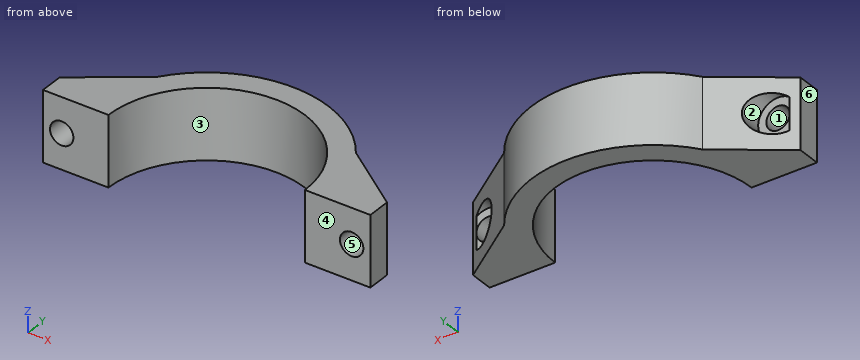
```python
from build123d import *

# Parameters (mm, degrees)
SALIENTE_EXTRUIR1_DEPTH = 7.5
SALIENTE_EXTRUIR2_DEPTH = 7.5
CROQUIS3_R              = 2.5
CORTAR_EXTRUIR1_DEPTH   = 45.240818256
CROQUIS4_R              = 4.25
CORTAR_EXTRUIR2_DEPTH   = 41.959224846


with BuildPart() as part:
    # Croquis1 → Saliente-Extruir1 (new, symmetric)
    with BuildSketch(Plane.XY):
        with BuildLine():
            Line((-26, 0), (-21, 0))
            ThreePointArc((-21, 0), (0, 21), (21, 0))
            Line((21, 0), (26, 0))
            ThreePointArc((26, 0), (0, 26), (-26, 0))
        make_face()
    extrude(amount=SALIENTE_EXTRUIR1_DEPTH, both=True)

    # Croquis2 → Saliente-Extruir2 (add, symmetric)
    with BuildSketch(Plane.XY):
        with BuildLine():
            Line((26, 0), (35, 0))
            Line((35, 0), (35, 5))
            Line((35, 5), (21.236760582, 15))
            ThreePointArc((21.236760582, 15), (24.78059498, 7.869060455), (26, 0))
        make_face()
    saliente_extruir2 = extrude(amount=SALIENTE_EXTRUIR2_DEPTH, both=True)

    # Croquis3 → Cortar-Extruir1 (cut, through all)
    with BuildSketch(Plane.XZ):
        with Locations(Location((31, 0, 0), (0, 0, 270))):
            Circle(CROQUIS3_R)
    cortar_extruir1 = extrude(amount=-CORTAR_EXTRUIR1_DEPTH, mode=Mode.SUBTRACT)

    # Croquis4 → Cortar-Extruir2 (cut, through all)
    with BuildSketch(Plane(origin=(0, 6.09, 0), x_dir=(-1, 0, 0), z_dir=(0, -1, 0))):
        with Locations((-31, 0)):
            Circle(CROQUIS4_R)
    cortar_extruir2 = extrude(amount=-CORTAR_EXTRUIR2_DEPTH, mode=Mode.SUBTRACT)

    # Simetría1: Saliente-Extruir2, Cortar-Extruir1, Cortar-Extruir2 across plane
    add(saliente_extruir2.mirror(Plane(origin=(0, 0, 0), x_dir=(0, 0, 1), z_dir=(1, 0, 0))))
    add(cortar_extruir1.mirror(Plane(origin=(0, 0, 0), x_dir=(0, 0, 1), z_dir=(1, 0, 0))), mode=Mode.SUBTRACT)
    add(cortar_extruir2.mirror(Plane(origin=(0, 0, 0), x_dir=(0, 0, 1), z_dir=(1, 0, 0))), mode=Mode.SUBTRACT)


solid = part.part
```
The listing builds one solid part. Answer for the finished solid, in the listing's coordinates (mm). Face numbers are marked on the shaded views. A direction names the side the tool comes from. Round coordinates to 2 decimals unless told otherwise and drop trailing zeros. Write each loop counter-clockwise with the first axis right and the second up, starting at its lowest first coordinate (ties: lowest second). Pieces come first, ordered by that corner, then holes. Notation, with made-up numbers: (83.5, 67.25) -> (122.5, 67.25) arc R26 ccw to (122.5, 104.25) -> close; hole circle Ø6 at (-20.5, -25.5). An arc over 180 degrees is marked (long way). Use CSV: the item, a comma, the result in double quotes. Start each with the question number.
(1) Section A-A on y = 13.25 is taken. Give the vertices of the cut face in (x, z), then the cut area to 3 significant figures.
(2) Which of the six approach directions +Z, -Z, +X, -X, +Y, -Y give full straight-line access (tool end or side, diameter ignored) to the marked faces 1 and 2?
(3) The mould has two halves that part along X. Classify the marked faces 3, 4, 5 and 6: released by +X, released by -X, zero draft, split by the parting line, or undercut.
(4) Consider L1, parallel to Z at x = -31, y = 3.75; L2, parallel to X at y = 2.75, z = 0; L3, parallel to X at y = 3.5, z = 0. Determine where each line is inside the solid, lowest interval first. Write a range as from..to.
(5) Each of these flat-tipped pins is pushed along its axis until it touches: pin 1 (1 mm diameter, centred on x = 7.5, z = 4, fed in from +Y); pin 2 (2 mm diameter, centred on x = 31.5, z = 2, fed in from +Y); pin 3 (4 mm diameter, centred on y = 23, z = 3.5, fed in from -X). Where does it stop, or does it pass through?
(6) Section C-C on x = 31 is taken. Give the vertices of the cut face in (y, z), then the cut area to 3 significant figures.
(7) Section B-B on z = 5.25 is taken. Give the vertices of the cut face in (x, y), then the cut area to 3 significant figures.
(8) Section D-D on y = 16.25 is taken. Give the vertices of the cut face in (x, z), then the cut area to 3 significant figures.
A:
1,outline,"(-23.65, -7.5) -> (-16.29, -7.5) -> (-16.29, 7.5) -> (-23.65, 7.5) -> close; (16.29, -7.5) -> (23.65, -7.5) -> (23.65, 7.5) -> (16.29, 7.5) -> close"
1,area,"221 mm²"
2,face 1,"+Y, -Y"
2,face 2,"+Y"
3,face 3,"undercut"
3,face 4,"zero draft"
3,face 5,"undercut"
3,face 6,"released by -X"
4,L1,"z = -7.5..-2.5, 2.5..7.5"
4,L2,"x = -35..-33.5, -28.5..-20.82, 20.82..28.5, 33.5..35"
4,L3,"x = -35..-33.5, -28.5..-20.71, 20.71..28.5, 33.5..35"
5,pin 1,"stops at y = 25.04"
5,pin 2,"stops at y = 6.09"
5,pin 3,"stops at x = -15.33"
6,outline,"(0, -7.5) -> (7.91, -7.5) -> (7.91, -4.25) -> (6.09, -4.25) -> (6.09, -2.5) -> (0, -2.5) -> close; (0, 2.5) -> (6.09, 2.5) -> (6.09, 4.25) -> (7.91, 4.25) -> (7.91, 7.5) -> (0, 7.5) -> close"
6,area,"72.7 mm²"
7,outline,"(-35, 0) -> (-21, 0) arc R21 cw to (21, 0) -> (35, 0) -> (35, 5) -> (21.24, 15) arc R26 ccw to (-21.24, 15) -> (-35, 5) -> close"
7,area,"547 mm²"
8,outline,"(-20.3, -7.5) -> (-13.3, -7.5) -> (-13.3, 7.5) -> (-20.3, 7.5) -> close; (13.3, -7.5) -> (20.3, -7.5) -> (20.3, 7.5) -> (13.3, 7.5) -> close"
8,area,"210 mm²"
